CAD build for the part. Positions are in the model's coordinates, mm. A direction names the side the tool comes from. Round coordinates to 2 decimals unless told otherwise and drop trailing zeros. Order: outer loops, then holes, each group sorted by start corner. A loop starts at its lowest first (then second) coordinate and runs counter-clockwise, first axis right, second up. Notation, with made-up numbers: M 46,87 L 70,87 A11 cw 70,91 Z; hole C 69,-22 d11. An arc over 180 degrees is marked long. Answer as CSV lines item,"result". Start each with the question number.
```python
from build123d import *

# Parameters (mm, degrees)
SKETCH1_R           = 30
SKETCH1_R_2         = 25
BOSS_EXTRUDE1_DEPTH = 15
SKETCH1_3_R         = 10
SKETCH1_3_R_2       = 5
BOSS_EXTRUDE2_DEPTH = 7.5
BOSS_EXTRUDE3_DEPTH = 2.5


with BuildPart() as part:
    # Sketch1 → Boss-Extrude1 (new, symmetric)
    with BuildSketch(Plane(origin=(0, 0, 0), x_dir=(1, 0, 0), z_dir=(0, 1, 0))):
        with Locations(Location((0, 0, 0), (0, 0, 270))):
            Circle(SKETCH1_R)
        with Locations(Location((0, 0, 0), (0, 0, 270))):
            Circle(SKETCH1_R_2, mode=Mode.SUBTRACT)
    extrude(amount=BOSS_EXTRUDE1_DEPTH, both=True)



with BuildPart() as body_2:
    # Sketch1_3 → Boss-Extrude2 (new, symmetric)
    with BuildSketch(Plane(origin=(0, 0, 0), x_dir=(1, 0, 0), z_dir=(0, 1, 0))):
        with Locations(Location((0, 0, 0), (0, 0, 270))):
            Circle(SKETCH1_3_R)
        with Locations(Location((0, 0, 0), (0, 0, 270))):
            Circle(SKETCH1_3_R_2, mode=Mode.SUBTRACT)
    extrude(amount=BOSS_EXTRUDE2_DEPTH, both=True)


with BuildPart() as part_1:
    add(part.part)

    add(body_2.part)  # Boss-Extrude3 merges body 2
    # Sketch1_4 → Boss-Extrude3 (add, symmetric)
    with BuildSketch(Plane(origin=(0, 0, 0), x_dir=(1, 0, 0), z_dir=(0, 1, 0))):
        with BuildLine():
            ThreePointArc((-5.833333333, 8.122328621), (0, 10), (5.833333333, 8.122328621))
            ThreePointArc((5.833333333, 8.122328621), (5.220486958, 8.833923416), (5, 9.746794345))
            Line((5, 9.746794345), (5, 21.9089023))
            ThreePointArc((5, 21.9089023), (5.820464351, 23.524048006), (7.608695652, 23.814024239))
            ThreePointArc((7.608695652, 23.814024239), (0, 25), (-7.608695652, 23.814024239))
            ThreePointArc((-7.608695652, 23.814024239), (-5.820464351, 23.524048006), (-5, 21.9089023))
            Line((-5, 21.9089023), (-5, 9.746794345))
            ThreePointArc((-5, 9.746794345), (-5.220486958, 8.833923416), (-5.833333333, 8.122328621))
        make_face()
        with BuildLine():
            Line((21.473665961, -6.624324131), (10.940971508, -0.543270153))
            ThreePointArc((10.940971508, -0.543270153), (10.260645572, 0.104112618), (9.95080959, 0.990650545))
            ThreePointArc((9.95080959, 0.990650545), (9.987694827, 0.49593553), (10, 0))
            ThreePointArc((10, 0), (8.40162968, -5.423340181), (4.117476257, -9.112979166))
            ThreePointArc((4.117476257, -9.112979166), (5.040158614, -8.938036034), (5.940971508, -9.203524191))
            Line((5.940971508, -9.203524191), (16.473665961, -15.284578169))
            ThreePointArc((16.473665961, -15.284578169), (17.462190998, -16.802693993), (16.819202132, -18.496335844))
            ThreePointArc((16.819202132, -18.496335844), (21.650635095, -12.5), (24.427897784, -5.317688395))
            ThreePointArc((24.427897784, -5.317688395), (23.282655349, -6.721354014), (21.473665961, -6.624324131))
        make_face()
        with BuildLine():
            ThreePointArc((-24.427897784, -5.317688395), (-21.650635095, -12.5), (-16.819202132, -18.496335844))
            ThreePointArc((-16.819202132, -18.496335844), (-17.462190998, -16.802693993), (-16.473665961, -15.284578169))
            Line((-16.473665961, -15.284578169), (-5.940971508, -9.203524191))
            ThreePointArc((-5.940971508, -9.203524191), (-5.040158614, -8.938036034), (-4.117476257, -9.112979166))
            ThreePointArc((-4.117476257, -9.112979166), (-8.660254038, -5), (-9.95080959, 0.990650545))
            ThreePointArc((-9.95080959, 0.990650545), (-10.260645572, 0.104112618), (-10.940971508, -0.543270153))
            Line((-10.940971508, -0.543270153), (-21.473665961, -6.624324131))
            ThreePointArc((-21.473665961, -6.624324131), (-23.282655349, -6.721354014), (-24.427897784, -5.317688395))
        make_face()
    extrude(amount=BOSS_EXTRUDE3_DEPTH, both=True)


solid = part_1.part
```
Q1. Mould opens along Z. For faces 5 (the flat face through (25, -15, -7)), 6 (the cylindrical face through (-10.25, 0.04, -0.12)), 7 (the cylindrical face through (1.32, 0.21, -29.97)) say: +Z half, -Z half, draft (parallel to the pull), parting line (faces both ways), or undercut.
Q2. Band-saw the part on B-B, the plane y = -5.5. Write the cut outline in (x, z), then the cut area to 3 significant figures.
Q3. Tool access for faces 1 (the cylindrical face through (-9.76, 0.11, -2.17)), 2 (the flat face through (-14, -2.5, 9)), 3 (the flat face through (-11.281, 0.035, 12.287)), 4 (the flat face through (5, 7.5, 2)): list every direction of +Z, -Z, +X, -X, +Y, -Y with a clear straight run to the whole face (end or side of a thin tool).
Q4. Probe line 1 along X through (y, z) = (-7.25, 0); line 2 along X through (y, z) = (-0.75, 0); line 3 along Z through (x, y) = (-16.5, -0.5). List the from-to ranges inside material, lowest first. Write a range as from..to.
Q5. Drop flat-ended pins along their axis: P1, Ø21.5, axis at x = 15, z = 10.5, coming from the +Y side; P2, Ø4, axis at y = 1, z = -14.5, coming from the +X side; P3, Ø10, axis at x = 0, z = -2, coming from the -Y side; P4, Ø2, axis at y = 9.5, z = 8.5, coming from the +X side. Give the stop position or say it passes through.
Q6. Band-saw the part on D-D, the plane z = -13.5. Write the cut outline in (x, y), then the cut area to 3 significant figures.
Q7. Band-saw the part on A-A, the plane x = 0. Write the cut outline in (y, z).
Q8. Band-saw the part on C-C, the plane z = -3. Write the cut outline in (x, y).
Answer:
1,face 5,"draft"
1,face 6,"undercut"
1,face 7,"parting line"
2,outline,"C 0,0 d60; C 0,0 d20; hole C 0,0 d50; hole C 0,0 d10"
2,area,"1,100 mm^2"
3,face 1,"none"
3,face 2,"-Y"
3,face 3,"+Y, -Y"
3,face 4,"+Y"
4,line 1,"x = -30..-25, -10..-5, 5..10, 25..30"
4,line 2,"x = -30..-25, -10.33..-5, 5..10.33, 25..30"
4,line 3,"z = -25.05..-18.78, 3.75..15.3, 18.78..25.05"
5,P1,"stops at y = 15"
5,P2,"stops at x = 27.27"
5,P3,"stops at y = -7.5"
5,P4,"stops at x = 29.05"
6,outline,"M -26.79,-15 L -21.04,-15 L -21.04,15 L -26.79,15 Z; M -5,-2.5 L 5,-2.5 L 5,2.5 L -5,2.5 Z; M 21.04,-15 L 26.79,-15 L 26.79,15 L 21.04,15 Z"
6,area,"395 mm^2"
7,outline,"M -15,-30 L 15,-30 L 15,-25 L 2.5,-25 L 2.5,-10 L 7.5,-10 L 7.5,-5 L -7.5,-5 L -7.5,-10 L -2.5,-10 L -2.5,-25 L -15,-25 Z; M -15,25 L 15,25 L 15,30 L -15,30 Z; M -7.5,5 L 7.5,5 L 7.5,10 L -7.5,10 Z"
8,outline,"M -29.85,-15 L -24.82,-15 L -24.82,15 L -29.85,15 Z; M -9.54,-7.5 L -4,-7.5 L -4,7.5 L -9.54,7.5 Z; M 4,-7.5 L 9.54,-7.5 L 9.54,7.5 L 4,7.5 Z; M 24.82,-15 L 29.85,-15 L 29.85,15 L 24.82,15 Z"
